Geometry: final body of the model. Coordinates: model frame, mm. Coordinates: 2 decimals unless noted, no trailing zeros. Write each loop counter-clockwise with the first axis right and the second up, starting at its lowest first coordinate (ties: lowest second). Pieces come first, ordered by that corner, then holes.
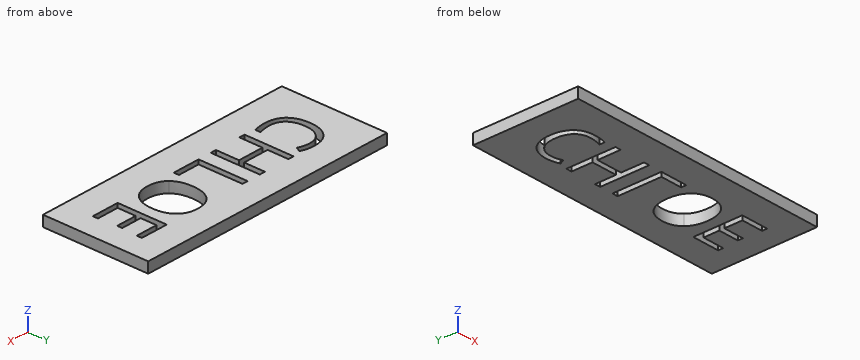
from build123d import *

# Parameters (mm, degrees)
F0_W     = 50
F0_H     = 20
F1_DEPTH = 2


with BuildPart() as f1:
    # F0 (on Top) → F1 (new body)
    with BuildSketch(Plane.XY):
        Rectangle(F0_W, F0_H)
        with BuildLine():
            add(Edge.make_bspline(
                [(-13.2876596552, 3.4753973501), (-14.3460879777, 3.970962056), (-15.4045163003, 3.970962056)],
                knots=[0, 0, 0, 1, 1, 1], degree=2))
            add(Edge.make_bspline(
                [(-15.4045163003, 3.970962056), (-16.9401550804, 3.970962056), (-17.8293164458, 2.9482225497)],
                knots=[0, 0, 0, 1, 1, 1], degree=2))
            add(Edge.make_bspline(
                [(-17.8293164458, 2.9482225497), (-18.7184778112, 1.9254830434), (-18.7184778112, 0.1471603126)],
                knots=[0, 0, 0, 1, 1, 1], degree=2))
            add(Edge.make_bspline(
                [(-18.7184778112, 0.1471603126), (-18.7184778112, -1.6801070805), (-17.8609265403, -2.6783742556)],
                knots=[0, 0, 0, 1, 1, 1], degree=2))
            add(Edge.make_bspline(
                [(-17.8609265403, -2.6783742556), (-17.0033752693, -3.6766414308), (-15.4167524659, -3.6766414308)],
                knots=[0, 0, 0, 1, 1, 1], degree=2))
            add(Edge.make_bspline(
                [(-15.4167524659, -3.6766414308), (-14.4419379414, -3.6766414308), (-13.1918096915, -3.3258713508)],
                knots=[0, 0, 0, 1, 1, 1], degree=2))
            Line((-13.1918096915, -3.3258713508), (-13.1918096915, -4.2741741832))
            add(Edge.make_bspline(
                [(-13.1918096915, -4.2741741832), (-14.1605061331, -4.6392197896), (-15.5819407012, -4.6392197896)],
                knots=[0, 0, 0, 1, 1, 1], degree=2))
            add(Edge.make_bspline(
                [(-15.5819407012, -4.6392197896), (-17.6396558794, -4.6392197896), (-18.7582453494, -3.3890915397)],
                knots=[0, 0, 0, 1, 1, 1], degree=2))
            add(Edge.make_bspline(
                [(-18.7582453494, -3.3890915397), (-19.8768348194, -2.1389632897), (-19.8768348194, 0.1614358391)],
                knots=[0, 0, 0, 1, 1, 1], degree=2))
            add(Edge.make_bspline(
                [(-19.8768348194, 0.1614358391), (-19.8768348194, 1.6012246556), (-19.3384435339, 2.6841253093)],
                knots=[0, 0, 0, 1, 1, 1], degree=2))
            add(Edge.make_bspline(
                [(-19.3384435339, 2.6841253093), (-18.8000522484, 3.767025963), (-17.7834308249, 4.3533422304)],
                knots=[0, 0, 0, 1, 1, 1], degree=2))
            add(Edge.make_bspline(
                [(-17.7834308249, 4.3533422304), (-16.7668094014, 4.9396584977), (-15.3902407738, 4.9396584977)],
                knots=[0, 0, 0, 1, 1, 1], degree=2))
            add(Edge.make_bspline(
                [(-15.3902407738, 4.9396584977), (-13.9259796262, 4.9396584977), (-12.828803446, 4.4053459341)],
                knots=[0, 0, 0, 1, 1, 1], degree=2))
            Line((-12.828803446, 4.4053459341), (-13.2876596552, 3.4753973501))
        make_face(mode=Mode.SUBTRACT)
        Polygon((-4.0840237789, 4.8071000372), (-4.0840237789, -4.510740051), (-5.1669244327, -4.510740051), (-5.1669244327, -0.126114052), (-10.0756661907, -0.126114052), (-10.0756661907, -4.510740051), (-11.1585668444, -4.510740051), (-11.1585668444, 4.8071000372), (-10.0756661907, 4.8071000372), (-10.0756661907, 0.8425823897), (-5.1669244327, 0.8425823897), (-5.1669244327, 4.8071000372), align=None, mode=Mode.SUBTRACT)
        Polygon((3.6655477543, -4.510740051), (-1.5287045339, -4.510740051), (-1.5287045339, 4.8071000372), (-0.4458038802, 4.8071000372), (-0.4458038802, -3.5298074438), (3.6655477543, -3.5298074438), align=None, mode=Mode.SUBTRACT)
        with BuildLine():
            add(Edge.make_bspline(
                [(12.2063913284, 3.6793334431), (13.3341579225, 2.4047328619), (13.3341579225, 0.1614358391)],
                knots=[0, 0, 0, 1, 1, 1], degree=2))
            add(Edge.make_bspline(
                [(13.3341579225, 0.1614358391), (13.3341579225, -2.0757431009), (12.2023126065, -3.3574814452)],
                knots=[0, 0, 0, 1, 1, 1], degree=2))
            add(Edge.make_bspline(
                [(12.2023126065, -3.3574814452), (11.0704672905, -4.6392197896), (9.0576180527, -4.6392197896)],
                knots=[0, 0, 0, 1, 1, 1], degree=2))
            add(Edge.make_bspline(
                [(9.0576180527, -4.6392197896), (6.9999028746, -4.6392197896), (5.8813134046, -3.3799144155)],
                knots=[0, 0, 0, 1, 1, 1], degree=2))
            add(Edge.make_bspline(
                [(5.8813134046, -3.3799144155), (4.7627239346, -2.1206090413), (4.7627239346, 0.1736720047)],
                knots=[0, 0, 0, 1, 1, 1], degree=2))
            add(Edge.make_bspline(
                [(4.7627239346, 0.1736720047), (4.7627239346, 2.4495988024), (5.884372446, 3.7017664133)],
                knots=[0, 0, 0, 1, 1, 1], degree=2))
            add(Edge.make_bspline(
                [(5.884372446, 3.7017664133), (7.0060209574, 4.9539340242), (9.0698542183, 4.9539340242)],
                knots=[0, 0, 0, 1, 1, 1], degree=2))
            add(Edge.make_bspline(
                [(9.0698542183, 4.9539340242), (11.0786247342, 4.9539340242), (12.2063913284, 3.6793334431)],
                knots=[0, 0, 0, 1, 1, 1], degree=2))
        make_face(mode=Mode.SUBTRACT)
        Polygon((20.6044796373, -3.5420436094), (20.6044796373, -4.510740051), (15.4102273491, -4.510740051), (15.4102273491, 4.8071000372), (20.6044796373, 4.8071000372), (20.6044796373, 3.8445216784), (16.4931280028, 3.8445216784), (16.4931280028, 0.8425823897), (20.3556776039, 0.8425823897), (20.3556776039, -0.1138778864), (16.4931280028, -0.1138778864), (16.4931280028, -3.5420436094), align=None, mode=Mode.SUBTRACT)
    extrude(amount=F1_DEPTH)


solid = f1.part
Item 1: Section A-A, the plane x = 18. Output: boundary loops of the cut face in (y, z).
Derived:
outline: (-10, 0) - (-4.51, 0) - (-4.51, 2) - (-10, 2) - close; (-3.54, 0) - (-0.11, 0) - (-0.11, 2) - (-3.54, 2) - close; (0.84, 0) - (3.84, 0) - (3.84, 2) - (0.84, 2) - close; (4.81, 0) - (10, 0) - (10, 2) - (4.81, 2) - close
Item 2: Pin query (flat end, axial travel): pin 1 (10 mm diameter, centred on x = -2, y = -4, fed in from -Z). Return the tip coordinate at first contact, or that it passes through.
Derived:
pin 1: stops at z = 0
Item 3: Section B-B, the plane z = 0.45. State how many separate pieces and enclosed holes the cut face has, plus the area to 3 significant figures.
Derived:
separate pieces: 1
enclosed holes: 5
area: 853 mm2
Item 4: Material intervals for probe 1 along X at (y, z) = (0, 0.5); probe 2 along Y at (x, z) = (19.5, 0.9); probe 3 along Y at (x, z) = (-9, 0.75), sorted ascending.
Derived:
probe 1: x = -25 to -19.88, -18.72 to -11.16, -4.08 to -1.53, -0.45 to 4.76, 13.33 to 15.41, 20.36 to 25
probe 2: y = -10 to -4.51, -3.54 to -0.11, 0.84 to 3.84, 4.81 to 10
probe 3: y = -10 to -0.13, 0.84 to 10
